from build123d import *

# Parameters (mm, degrees)
SKETCH1_W                 = 194
SKETCH1_H                 = 52
BOSS_EXTRUDE1_DEPTH       = 84
SKETCH2_W                 = 190
SKETCH2_H                 = 80
CUT_EXTRUDE1_DEPTH        = 50
FILLET1_R                 = 1
FILLET2_R                 = 1
FILLET3_R                 = 1
FILLET4_R                 = 3
FILLET5_R                 = 3
SKETCH3_W                 = 25
SKETCH3_H                 = 10
CUT_EXTRUDE2_DEPTH        = 5
F_4_0MM_DOWEL_HOLE1_D     = 4
F_4_0MM_DOWEL_HOLE1_DEPTH = 20
F_4_0MM_DOWEL_HOLE1_TIP   = 1.201721238
F_4_0MM_DOWEL_HOLE2_D     = 4
F_4_0MM_DOWEL_HOLE2_DEPTH = 20
F_4_0MM_DOWEL_HOLE2_TIP   = 1.201721238


with BuildPart() as part:
    # Sketch1 → Boss-Extrude1 (new body)
    with BuildSketch(Plane.XY):
        with Locations((97, 26)):
            Rectangle(SKETCH1_W, SKETCH1_H)
    extrude(amount=BOSS_EXTRUDE1_DEPTH)

    # Sketch2 → Cut-Extrude1 (cut)
    with BuildSketch(Plane.XZ):
        with Locations((97, 42)):
            Rectangle(SKETCH2_W, SKETCH2_H)
    extrude(amount=-CUT_EXTRUDE1_DEPTH, mode=Mode.SUBTRACT)

    # Fillet1
    fillet1_edges = [part.edges().sort_by_distance(p)[0] for p in [
        (97, 50, 2),
        (2, 50, 42),
        (2, 25, 2),
    ]]
    fillet(fillet1_edges, radius=FILLET1_R)

    # Fillet2
    fillet2_edges = [part.edges().sort_by_distance(p)[0] for p in [
        (97.5, 50, 82),
        (2, 24.5, 82),
        (2.292893219, 49.707106781, 82),
    ]]
    fillet(fillet2_edges, radius=FILLET2_R)

    # Fillet3
    fillet3_edges = [part.edges().sort_by_distance(p)[0] for p in [
        (192, 50, 42),
        (192, 24.5, 2),
        (192, 49.707106781, 2.292893219),
        (192, 24.5, 82),
        (192, 49.707106781, 81.707106781),
    ]]
    fillet(fillet3_edges, radius=FILLET3_R)

    # Fillet4
    fillet4_edges = [part.edges().sort_by_distance(p)[0] for p in [
        (194, 26, 84),
        (97, 52, 84),
        (0, 26, 84),
        (194, 52, 42),
    ]]
    fillet(fillet4_edges, radius=FILLET4_R)

    # Fillet5
    # the kernel refuses this fillet: 3 mm, written as the material it takes off along each edge
    with BuildSketch(Plane(origin=(3, 49, 81), x_dir=(0, 1, 0), z_dir=(-1, 0, 0))) as fillet5_piece_1_section:
        Polygon((0, 0), (FILLET5_R, 0), (FILLET5_R, -FILLET5_R), (0, -FILLET5_R), align=None)
    fillet5_piece_1 = extrude(amount=FILLET5_R, mode=Mode.PRIVATE)
    fillet5_piece_1 = fillet5_piece_1 - Plane(origin=(3, 49, 81), x_dir=(0, -0.7071067811865475, -0.7071067811865475), z_dir=(-1, 0, 0)) * Sphere(FILLET5_R, mode=Mode.PRIVATE)
    add(fillet5_piece_1, mode=Mode.SUBTRACT)
    with BuildSketch(Plane(origin=(3, 49, 3), x_dir=(0, 0, -1), z_dir=(-1, 0, 0))) as fillet5_piece_2_section:
        Polygon((0, 0), (FILLET5_R, 0), (FILLET5_R, -FILLET5_R), (0, -FILLET5_R), align=None)
    fillet5_piece_2 = extrude(amount=FILLET5_R, mode=Mode.PRIVATE)
    fillet5_piece_2 = fillet5_piece_2 - Plane(origin=(3, 49, 3), x_dir=(0, -0.7071067811865475, 0.7071067811865475), z_dir=(-1, 0, 0)) * Sphere(FILLET5_R, mode=Mode.PRIVATE)
    add(fillet5_piece_2, mode=Mode.SUBTRACT)
    with BuildSketch(Plane(origin=(194, -7.5, 0), x_dir=(-1, 0, 0), z_dir=(0, 1, 0))) as fillet5_piece_3:
        with BuildLine():
            CenterArc((FILLET5_R, FILLET5_R), FILLET5_R, 180, 90)
            Line((0, FILLET5_R), (0, 0))
            Line((0, 0), (FILLET5_R, 0))
        make_face()
    extrude(amount=56.5, mode=Mode.SUBTRACT)
    with BuildSketch(Plane(origin=(0, 49, 0), x_dir=(0, 0, 1), z_dir=(0, -1, 0))) as fillet5_piece_4:
        with BuildLine():
            CenterArc((FILLET5_R, -FILLET5_R), FILLET5_R, 90, 90)
            Line((0, -FILLET5_R), (0, 0))
            Line((0, 0), (FILLET5_R, 0))
        make_face()
    extrude(amount=56.5, mode=Mode.SUBTRACT)
    with BuildSketch(Plane(origin=(191, 52, 0), x_dir=(0, -1, 0), z_dir=(-1, 0, 0))) as fillet5_piece_5:
        with BuildLine():
            CenterArc((FILLET5_R, FILLET5_R), FILLET5_R, 180, 90)
            Line((0, FILLET5_R), (0, 0))
            Line((0, 0), (FILLET5_R, 0))
        make_face()
    extrude(amount=188, mode=Mode.SUBTRACT)
    with BuildSketch(Plane(origin=(0, 52, 3), x_dir=(0, -1, 0), z_dir=(0, 0, 1))) as fillet5_piece_6:
        with BuildLine():
            CenterArc((FILLET5_R, FILLET5_R), FILLET5_R, 180, 90)
            Line((0, FILLET5_R), (0, 0))
            Line((0, 0), (FILLET5_R, 0))
        make_face()
    extrude(amount=78, mode=Mode.SUBTRACT)
    with BuildSketch(Plane(origin=(191, 49, 0), x_dir=(1, 0, 0), z_dir=(0, -1, 0))) as fillet5_piece_7:
        with BuildLine():
            CenterArc((3 - FILLET5_R, FILLET5_R), FILLET5_R, 270, 90)
            Line((3, FILLET5_R), (3, 0))
            Line((3, 0), (3 - FILLET5_R, 0))
        make_face()
    revolve(axis=Axis((191, 49, 0), (0, 0, 1)), revolution_arc=90, mode=Mode.SUBTRACT)

    # Sketch3 → Cut-Extrude2 (cut)
    with BuildSketch(Plane(origin=(194, 0, 0), x_dir=(0, 0, -1), z_dir=(1, 0, 0))):
        with Locations((-69.5, 5)):
            Rectangle(SKETCH3_W, SKETCH3_H)
    extrude(amount=-CUT_EXTRUDE2_DEPTH, mode=Mode.SUBTRACT)

    # Ø4.0mm Dowel Hole1
    with Locations(Plane(origin=(194, 5, 42.107279869), x_dir=(0, 0, 1), z_dir=(1, 0, 0))):
        with Locations((0, 0)):
            Hole(F_4_0MM_DOWEL_HOLE1_D / 2, depth=F_4_0MM_DOWEL_HOLE1_DEPTH)
            with Locations((0, 0, -(F_4_0MM_DOWEL_HOLE1_DEPTH + F_4_0MM_DOWEL_HOLE1_TIP / 2))):  # 118° drill point
                Cone(0, F_4_0MM_DOWEL_HOLE1_D / 2, F_4_0MM_DOWEL_HOLE1_TIP, mode=Mode.SUBTRACT)

    # Ø4.0mm Dowel Hole2
    with Locations(Plane(origin=(0, 5, 41.892720131), x_dir=(0, 0, -1), z_dir=(-1, 0, 0))):
        with Locations((0, 0)):
            Hole(F_4_0MM_DOWEL_HOLE2_D / 2, depth=F_4_0MM_DOWEL_HOLE2_DEPTH)
            with Locations((0, 0, -(F_4_0MM_DOWEL_HOLE2_DEPTH + F_4_0MM_DOWEL_HOLE2_TIP / 2))):  # 118° drill point
                Cone(0, F_4_0MM_DOWEL_HOLE2_D / 2, F_4_0MM_DOWEL_HOLE2_TIP, mode=Mode.SUBTRACT)


solid = part.part
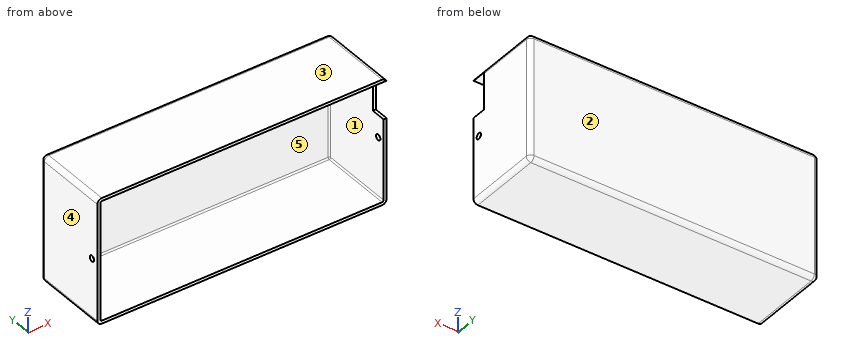
Read the model definition and answer for the solid it produces. Units are mm, in the model's axes. Face numbers are marked on the shaded views. A direction names the side the tool comes from. Coordinates: 2 decimals unless noted, no trailing zeros. Loops run counter-clockwise (first coordinate to the right, second up) from the corner with the lowest first, then second, coordinate; pieces in that order, holes last. Notation, with made-up numbers: (39.25, -9) -> (77.25, -9) arc R26 ccw to (77.25, 24) -> close; hole circle Ø11 at (6.25, 72). An arc over 180 degrees is marked (long way). Answer in a Markdown table with one row per item.
Item 1: A cutting plane is placed at A-A on y = 19. Determine the outline of the cut face in (x, z), plus the area to 3 significant figures.
Returned:
| item | result |
|---|---|
| outline | (0, 3) arc R3 ccw to (3, 0) -> (191, 0) arc R3 ccw to (194, 3) -> (194, 81) arc R3 ccw to (191, 84) -> (3, 84) arc R3 ccw to (0, 81) -> close; hole (2, 3) arc R1 ccw to (3, 2) -> (191, 2) arc R1 ccw to (192, 3) -> (192, 81) arc R1 ccw to (191, 82) -> (3, 82) arc R1 ccw to (2, 81) -> close |
| area | 1,090 mm^2 |
Item 2: A cutting plane is placed at B-B on y = 5. Determine the outline of the cut face in (x, z).
Returned:
| item | result |
|---|---|
| outline | (0, 3) arc R3 ccw to (3, 0) -> (191, 0) arc R3 ccw to (194, 3) -> (194, 40.11) -> (192, 40.11) -> (192, 3) arc R1 cw to (191, 2) -> (3, 2) arc R1 cw to (2, 3) -> (2, 39.89) -> (0, 39.89) -> close; (0, 43.89) -> (2, 43.89) -> (2, 81) arc R1 cw to (3, 82) -> (193.83, 82) arc R3 ccw to (191, 84) -> (3, 84) arc R3 ccw to (0, 81) -> close; (192, 44.11) -> (194, 44.11) -> (194, 57) -> (192, 57) -> close |
Item 3: For a pull along Z with two mould halves and no side action, classify the marked faces 3, 4 and 5 as released by +Z, released by -Z, zero draft, split by the parting line, or undercut.
Returned:
| item | result |
|---|---|
| face 3 | released by +Z |
| face 4 | zero draft |
| face 5 | undercut |
Item 4: Straight lines are drawn through the part: line 1 along Z through (x, y) = (13, 24.5); line 2 along X through (y, z) = (43.5, 63.5); line 3 along Y through (x, z) = (169.5, 57). For each, find the intervals that lie inside material, in ascending order. Write a range as [from, to].
Returned:
| item | result |
|---|---|
| line 1 | z = [0, 2], [82, 84] |
| line 2 | x = [0, 2], [192, 194] |
| line 3 | y = [50, 52] |
Item 5: Each of these flat-tipped pins is pushed along its axis until it touches: P1, Ø12, axis at x = 170.5, z = 70, coming from the -Y side; P2, Ø1, axis at x = 193, y = 6, coming from the +Z side; P3, Ø0.9, axis at x = 192.5, z = 69, coming from the -Y side. Where does it stop, or does it pass through?
Returned:
| item | result |
|---|---|
| P1 | stops at y = 50 |
| P2 | stops at z = 83.6 |
| P3 | stops at y = 10 |
Item 6: A cutting plane is placed at C-C on x = 137. Determine the outline of the cut face in (y, z), plus the area to 3 significant figures.
Returned:
| item | result |
|---|---|
| outline | (0, 0) -> (49, 0) arc R3 ccw to (52, 3) -> (52, 81) arc R3 ccw to (49, 84) -> (0, 84) -> (0, 82) -> (49, 82) arc R1 cw to (50, 81) -> (50, 3) arc R1 cw to (49, 2) -> (0, 2) -> close |
| area | 365 mm^2 |
Item 7: For the marked faces 1 and 2, determine the directions among +Z, -Z, +X, -X, +Y, -Y from which every point of the face is accessible in a straight line to the end or side of a thin tool.
Returned:
| item | result |
|---|---|
| face 1 | -Y |
| face 2 | +Z, -Z, +X, -X, +Y |
Item 8: A cutting plane is placed at D-D on z = 11. Determine the outline of the cut face in (x, y).
Returned:
| item | result |
|---|---|
| outline | (0, 0) -> (2, 0) -> (2, 49) arc R1 cw to (3, 50) -> (191, 50) arc R1 cw to (192, 49) -> (192, 0) -> (194, 0) -> (194, 49) arc R3 ccw to (191, 52) -> (3, 52) arc R3 ccw to (0, 49) -> close |
